from build123d import *

# Parameters (mm, degrees)
SCHIZZO1_W                   = 28
SCHIZZO1_H                   = 25
ESTRUSIONE_ESTRUSIONE1_DEPTH = 1.2
SCHIZZO4_W                   = 22
SCHIZZO4_H                   = 21
TAGLIO_ESTRUSIONE1_DEPTH     = 19.806647761
SCHIZZO2_R                   = 1.75
ESTRUSIONE_ESTRUSIONE2_DEPTH = 2.4
ESTRUSIONE_ESTRUSIONE3_DEPTH = 23.146699141
SCHIZZO5_W                   = 28
SCHIZZO5_H                   = 4
ESTRUSIONE_ESTRUSIONE4_DEPTH = 2.3


with BuildPart() as part:
    # Schizzo1 → Estrusione-Estrusione1 (new body)
    with BuildSketch(Plane.XY):
        Rectangle(SCHIZZO1_W, SCHIZZO1_H)
    extrude(amount=ESTRUSIONE_ESTRUSIONE1_DEPTH)

    # Schizzo4 → Taglio-Estrusione1 (cut, through all)
    with BuildSketch(Plane.XY.offset(1.2)):
        with Locations((0, 2)):
            Rectangle(SCHIZZO4_W, SCHIZZO4_H)
    extrude(amount=-TAGLIO_ESTRUSIONE1_DEPTH, mode=Mode.SUBTRACT)

    # Schizzo2 → Estrusione-Estrusione2 (add)
    with BuildSketch(Plane(origin=(14, 0, 0), x_dir=(0, 0, -1), z_dir=(1, 0, 0))):
        with BuildLine():
            Line((0, -12.5), (0, -16.5))
            ThreePointArc((0, -16.5), (-5.185062871, -19.964548247), (-6.401650429, -13.848349571))
            Line((-6.401650429, -13.848349571), (-3.2, -10.646699141))
            Line((-3.2, -10.646699141), (-1.2, -10.646699141))
            Line((-1.2, -10.646699141), (-1.2, -12.5))
            Line((-1.2, -12.5), (0, -12.5))
        make_face()
        with Locations((-3.75, -16.5)):
            Circle(SCHIZZO2_R, mode=Mode.SUBTRACT)
    estrusione_estrusione2 = extrude(amount=-ESTRUSIONE_ESTRUSIONE2_DEPTH)

    # Schizzo3 → Estrusione-Estrusione3 (add)
    with BuildSketch(Plane(origin=(0, 12.5, 0), x_dir=(1, 0, 0), z_dir=(0, 1, 0))):
        Polygon((14, -1.2), (14, -3.5), (11.6, -3.5), (11.6, -2.3), (12.8, -2.3), (12.8, -1.2), align=None)
    estrusione_estrusione3 = extrude(amount=-ESTRUSIONE_ESTRUSIONE3_DEPTH)

    # Specchia1: Estrusione-Estrusione2, Estrusione-Estrusione3 across plane
    add(estrusione_estrusione2.mirror(Plane(origin=(0, 0, 0), x_dir=(0, 0, 1), z_dir=(1, 0, 0))))
    add(estrusione_estrusione3.mirror(Plane(origin=(0, 0, 0), x_dir=(0, 0, 1), z_dir=(1, 0, 0))))

    # Schizzo5 → Estrusione-Estrusione4 (add)
    with BuildSketch(Plane.XY.offset(1.2)):
        with Locations((0, -10.5)):
            Rectangle(SCHIZZO5_W, SCHIZZO5_H)
    extrude(amount=ESTRUSIONE_ESTRUSIONE4_DEPTH)


solid = part.part
Design review of the part built by this model. Coordinates are the model's own, in mm. A direction names the side the tool comes from. Coordinates: 2 decimals unless noted, no trailing zeros. Write each loop counter-clockwise with the first axis right and the second up, starting at its lowest first coordinate (ties: lowest second). Pieces come first, ordered by that corner, then holes. Notation, with made-up numbers: (55, -27) -> (110, -27) arc R27 ccw to (110, 9) -> close; hole circle Ø3 at (-25.75, 49.25). An arc over 180 degrees is marked (long way). Write each question's results on one line, items separated by ' | '. Start each with the question number.
(1) Tool access review of faces 1 (the face through (11.6, 2, 3)), 2 (the face through (-11, 2, 1)), 3 (the face through (-14, -7, 2)), 4 (the face through (12, 2, 1.2)), 5 (the face through (14, -4, 2)): name each direction out of +Z, -Z, +X, -X, +Y, -Y from which nothing blocks a thin tool from reaching the whole face with its end or side.
(2) Take a section at B-B on y = 7. Write out the cut boundary in (x, z).
(3) For line 1 along X through (y, z) = (-2, 2.75); line 2 along X through (y, z) = (-5.5, 1.75); line 3 along Y through (x, z) = (10.5, 3.25), list the stretches that pass through material, from the lowest coordinate up. Write a range as from..to.
(4) Take a section at D-D on z = 4.25. Write out the cut boundary in (x, y), and give its area (3 significant figures).
(5) Clearance check with flat-ended pins moving along their axes: P1, Ø0.5, axis at x = 12, y = -2.5, coming from the +Z side; P2, Ø4, axis at x = 4, z = 1, coming from the -Y side; P3, Ø1.5, axis at x = 5.5, z = 4, coming from the +Y side. State where each tip first meets the part, or that it passes through.
(6) Take a section at A-A on z = 7. Write out the cut boundary in (x, y), and give its area (3 significant figures).
(7) The part is to be moulded in two halves that separate along Y. For faces 6 (the face through (-13, 12.5, 2)), 7 (the face through (12.817, -14.765, 3.978)), 8 (the face through (-12, 2, 2.3)), say which applies: pulls with the +Y half, pulls with the -Y half, needs draft (parallel to the pull), parting line crosses it, or undercut.
(8) Take a section at C-C on z = 0.75. Write out the cut boundary in (x, y), and give its area (3 significant figures).
Results found:
1) face 1: +Z, +Y | face 2: +Z, -Z, +Y | face 3: +Z, -Z, -X, +Y, -Y | face 4: +Y | face 5: +Z, -Z, +X, +Y, -Y
2) outline: (-14, 0) -> (-11, 0) -> (-11, 1.2) -> (-12.8, 1.2) -> (-12.8, 2.3) -> (-11.6, 2.3) -> (-11.6, 3.5) -> (-14, 3.5) -> close; (11, 0) -> (14, 0) -> (14, 3.5) -> (11.6, 3.5) -> (11.6, 2.3) -> (12.8, 2.3) -> (12.8, 1.2) -> (11, 1.2) -> close
3) line 1: x = -14..-11.6, 11.6..14 | line 2: x = -14..-12.8, 12.8..14 | line 3: y = -12.5..-8.5
4) outline: (-14, -20.22) -> (-11.6, -20.22) -> (-11.6, -18.18) -> (-14, -18.18) -> close; (-14, -14.82) -> (-11.6, -14.82) -> (-11.6, -11.7) -> (-14, -11.7) -> close; (11.6, -20.22) -> (14, -20.22) -> (14, -18.18) -> (11.6, -18.18) -> close; (11.6, -14.82) -> (14, -14.82) -> (14, -11.7) -> (11.6, -11.7) -> close | area: 24.8 mm2
5) P1: stops at z = 3.5 | P2: stops at y = -12.5 | P3: stops at y = -8.5
6) outline: (-14, -18.37) -> (-11.6, -18.37) -> (-11.6, -14.63) -> (-14, -14.63) -> close; (11.6, -18.37) -> (14, -18.37) -> (14, -14.63) -> (11.6, -14.63) -> close | area: 18.0 mm2
7) face 6: pulls with the +Y half | face 7: undercut | face 8: needs draft
8) outline: (-14, -18.75) -> (-11.6, -18.75) -> (-11.6, -12.5) -> (11.6, -12.5) -> (11.6, -18.75) -> (14, -18.75) -> (14, 12.5) -> (11, 12.5) -> (11, -8.5) -> (-11, -8.5) -> (-11, 12.5) -> (-14, 12.5) -> close | area: 268 mm2
